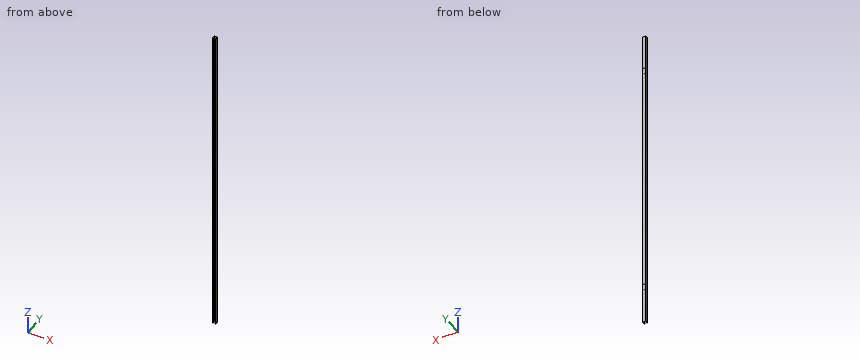
from build123d import *

# Parameters (mm, degrees)
F1_DEPTH    = 450
F2_T1_DEPTH = 452.5
F2_T3_DEPTH = 7.2
F3_R        = 0.5
F4_DEPTH    = 25


# Not quite as in the source:
# - a fillet or chamfer that OpenCascade refuses, or shapes differently, is made with other operations: its cross-section is extruded or revolved along the edge and cut away or added


with BuildPart() as f1:
    # F0 (on Top) → F1 (new body)
    with BuildSketch(Plane.XY):
        Polygon((-3.0933290763, 0), (-1.5933290763, 0), (-1.5933290763, 0.3), (-2.7933290763, 0.3), (-2.7933290763, 4.4), (1.6066709237, 4.4), (1.6066709237, 0.3), (0.4066709237, 0.3), (0.4066709237, 0), (1.9066709237, 0), (1.9066709237, 4.7), (-3.0933290763, 4.7), align=None)
    extrude(amount=F1_DEPTH)

    # F2: fillet of radius 0.5 on 8 edges, made by hand

    # F2_s2 → F2_t1 (cut)
    with BuildSketch(Plane.XY.offset(-1.25)):
        with BuildLine():
            ThreePointArc((-3.0933290763, 4.2), (-2.9468824669, 4.5535533906), (-2.5933290763, 4.7))
            Line((-2.5933290763, 4.7), (-3.0933290763, 4.7))
            Line((-3.0933290763, 4.7), (-3.0933290763, 4.2))
        make_face()
        with BuildLine():
            ThreePointArc((-3.0933290763, 0.5), (-2.9468824669, 0.1464466094), (-2.5933290763, 0))
            Line((-2.5933290763, 0), (-3.0933290763, 0))
            Line((-3.0933290763, 0), (-3.0933290763, 0.5))
        make_face()
        with BuildLine():
            ThreePointArc((1.4066709237, 0), (1.7602243143, 0.1464466094), (1.9066709237, 0.5))
            Line((1.9066709237, 0.5), (1.9066709237, 0))
            Line((1.9066709237, 0), (1.4066709237, 0))
        make_face()
        with BuildLine():
            ThreePointArc((1.9066709237, 4.2), (1.7602243143, 4.5535533906), (1.4066709237, 4.7))
            Line((1.4066709237, 4.7), (1.9066709237, 4.7))
            Line((1.9066709237, 4.7), (1.9066709237, 4.2))
        make_face()
    extrude(amount=F2_T1_DEPTH, mode=Mode.SUBTRACT)

    # F2_s4 → F2_t3 (cut)
    with BuildSketch(Plane.XZ.offset(-5.95)):
        with BuildLine():
            ThreePointArc((-3.0933290763, 0.5), (-2.9468824669, 0.1464466094), (-2.5933290763, 0))
            Line((-2.5933290763, 0), (-3.0933290763, 0))
            Line((-3.0933290763, 0), (-3.0933290763, 0.5))
        make_face()
        with BuildLine():
            ThreePointArc((-3.0933290763, 449.5), (-2.9468824669, 449.8535533906), (-2.5933290763, 450))
            Line((-2.5933290763, 450), (-3.0933290763, 450))
            Line((-3.0933290763, 450), (-3.0933290763, 449.5))
        make_face()
        with BuildLine():
            ThreePointArc((1.9066709237, 0.5), (1.7602243143, 0.1464466094), (1.4066709237, 0))
            Line((1.4066709237, 0), (1.9066709237, 0))
            Line((1.9066709237, 0), (1.9066709237, 0.5))
        make_face()
        with BuildLine():
            ThreePointArc((1.9066709237, 449.5), (1.7602243143, 449.8535533906), (1.4066709237, 450))
            Line((1.4066709237, 450), (1.9066709237, 450))
            Line((1.9066709237, 450), (1.9066709237, 449.5))
        make_face()
    extrude(amount=F2_T3_DEPTH, mode=Mode.SUBTRACT)

    # F3 (on face) → F4 (cut)
    with BuildSketch(Plane(origin=(0, 4.7, 0), x_dir=(-1, 0, 0), z_dir=(0, 1, 0))):
        with Locations((0.5933290763, 400)):
            Circle(F3_R)
        with Locations((0.5933290763, 391)):
            Circle(F3_R)
        with Locations((0.5933290763, 50)):
            Circle(F3_R)
        with Locations((0.5933290763, 59)):
            Circle(F3_R)
    extrude(amount=-F4_DEPTH, mode=Mode.SUBTRACT)


solid = f1.part
Check sheet for the modelled part. Datum: model origin and axes. Units: mm. Give positions to 0.01 mm unless a question says otherwise; leave off trailing zeros. Loops run counter-clockwise (first coordinate to the right, second up) from the corner with the lowest first, then second, coordinate; pieces in that order, holes last. Notation, with made-up numbers: M -11.5,48 L 2.5,48 A20 ccw 2.5,72 Z; hole C 29,-40 d4. An arc over 180 degrees is marked long. Use a Markdown table: item, result. Add a question column.
Q1. Scan lines: line 1 along X through (y, z) = (1.6, 291); line 2 along Y through (x, z) = (0.55, 415.5); line 3 along Y through (x, z) = (-0.05, 67.5). Record each from-to range of solid material in increasing order. Write a range as [from, to].
Q2. Sectioned sample at B-B, the plane z = 306.5. Record the cut outline in (x, y).
Q3. Sectioned sample at A-A, the plane y = 1.9. Record the cut outline in (x, z).
Q4. Go/stop test with flat-tipped pins: pin 1 (2 mm diameter, centred on x = -0.5, y = 1, fed in from -Z); pin 2 (3 mm diameter, centred on x = 0.5, z = 265.5, fed in from -Y). Record where each tip stops, or that it passes through.
Verdict:
| question | item | result |
|---|---|---|
| 1 | line 1 | [-3.09, -2.79], [1.61, 1.91] |
| 1 | line 2 | [0, 0.3], [4.4, 4.7] |
| 1 | line 3 | [4.4, 4.7] |
| 2 | outline | M -3.09,0.5 A0.5 ccw -2.59,0 L -1.59,0 L -1.59,0.3 L -2.79,0.3 L -2.79,4.4 L 1.61,4.4 L 1.61,0.3 L 0.41,0.3 L 0.41,0 L 1.41,0 A0.5 ccw 1.91,0.5 L 1.91,4.2 A0.5 ccw 1.41,4.7 L -2.59,4.7 A0.5 ccw -3.09,4.2 Z |
| 3 | outline | M -3.09,0.5 A0.5 ccw -2.79,0.04 L -2.79,449.96 A0.5 ccw -3.09,449.5 Z; M 1.61,0.04 A0.5 ccw 1.91,0.5 L 1.91,449.5 A0.5 ccw 1.61,449.96 Z |
| 4 | pin 1 | through |
| 4 | pin 2 | y = 0 |
